Could you check a few things on this drawing? It's one solid part, dimensions in mm from its lowest x, y, z. A direction names the side the tool comes from. Give positions to 0.01 mm unless a question says otherwise; leave off trailing zeros. Loops run counter-clockwise (first coordinate to the right, second up) from the corner with the lowest first, then second, coordinate; pieces in that order, holes last.
Q1. Suppose I cut it at A-A (z = 27.5). List the corners of the cut face in (x, y) for me (1 decimal), and give its area (3 significant figures).
Q2. Suppose I cut it at D-D (y = 12). List the corners of the cut face in (x, z) for me.
Q3. For the marked faces 5 and 6, which set-ups out of +Z, -Z, +X, -X, +Y, -Y let a thin tool reach every point of the face, with its end or its side?
Q4. Thinking about a two-plate mould opening in Z: for the marked faces 1, 2, 3 and 4, which applies, pulls with the +Z half, pulls with the -Z half, needs draft (parallel to the pull), parting line crosses it, or undercut?
Q5. I'm going to push flat-ended pins straight in: P1, Ø3, axis at y = 53.315, z = 27.5, coming from the +X side; P2, Ø22.5, axis at y = 39.5, z = 20.5, coming from the +X side; P3, Ø11.5, axis at x = 34, z = 35.5, coming from the +Y side (3 decimals); P4, Ø6, axis at y = 17, z = 43.5, coming from the -X side. Where does each tip first touch, or does it pass through?
Q6. I need wall thicknesses on probe 1 along Z at (x, y) = (31, 9); probe 2 along Y at (x, z) = (2, 27) (1 decimal); probe 3 along X at (y, z) = (25, 26). Which ranges of each line are inside material? Lowest first, please.
Q7. Suppose I cut it at C-C (x = 34). List the corners of the cut face in (y, z) for me (1 decimal).
Q8. Suppose I cut it at B-B (z = 22). List the corners of the cut face in (x, y) for me (1 decimal).
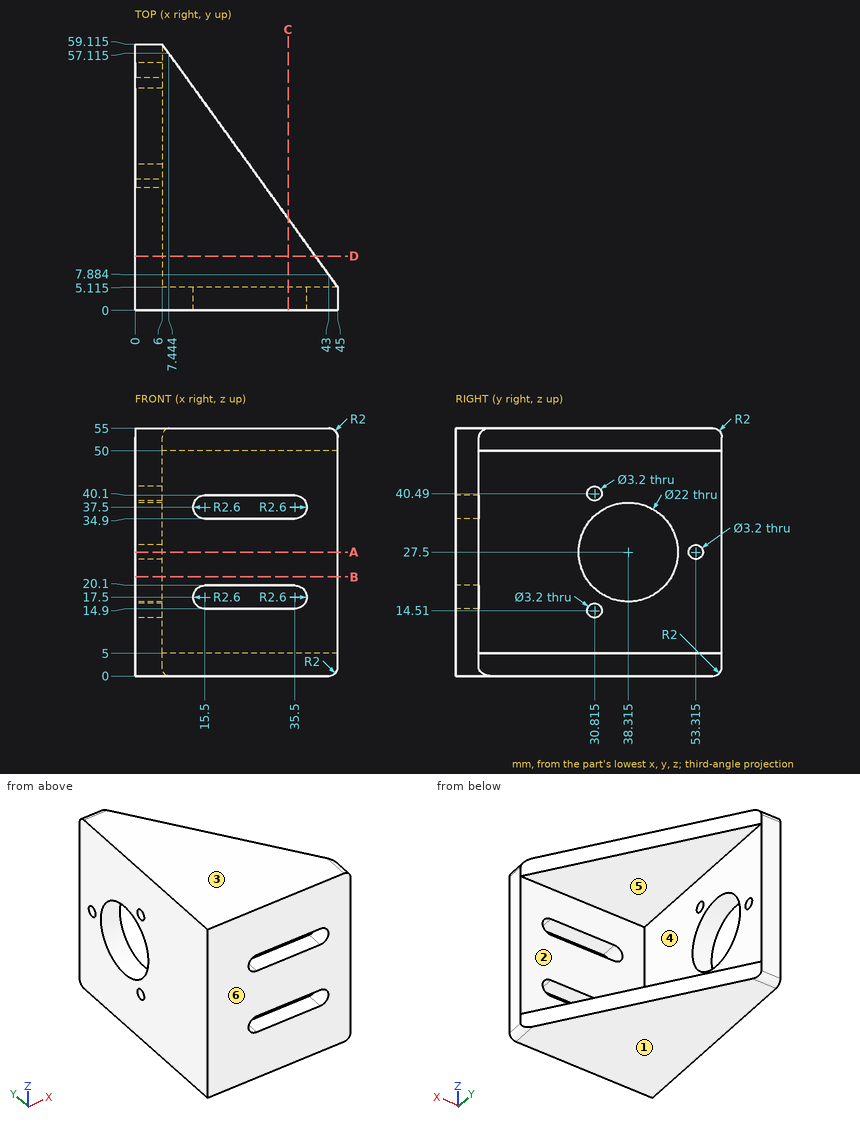
Solutions:
1. outline: (0, 0) - (45, 0) - (45, 5.1) - (6, 5.1) - (6, 27.3) - (0, 27.3) - close; (0, 49.3) - (6, 49.3) - (6, 51.7) - (0, 51.7) - close; (0, 54.9) - (6, 54.9) - (6, 59.1) - (0, 59.1) - close
1. area: 403 mm2
2. outline: (0, 0) - (40.03, 0) - (40.03, 5) - (6, 5) - (6, 50) - (40.03, 50) - (40.03, 55) - (0, 55) - close
3. face 5: +X, +Y
3. face 6: +Z, -Z, +X, -X, -Y
4. face 1: pulls with the -Z half
4. face 2: undercut
4. face 3: pulls with the +Z half
4. face 4: undercut
5. P1: passes through
5. P2: stops at x = 6
5. P3: stops at y = 5.115
5. P4: stops at x = 0
6. probe 1: z = 0 to 5, 50 to 55
6. probe 2: y = 0 to 27.3, 49.3 to 51.8, 54.8 to 59.1
6. probe 3: x = 0 to 6
7. outline: (0, 0) - (20.3, 0) - (20.3, 5) - (5.1, 5) - (5.1, 14.9) - (0, 14.9) - close; (0, 20.1) - (5.1, 20.1) - (5.1, 34.9) - (0, 34.9) - close; (0, 40.1) - (5.1, 40.1) - (5.1, 50) - (20.3, 50) - (20.3, 55) - (0, 55) - close
8. outline: (0, 0) - (45, 0) - (45, 5.1) - (6, 5.1) - (6, 28.8) - (0, 28.8) - close; (0, 47.8) - (6, 47.8) - (6, 59.1) - (0, 59.1) - close
